from build123d import *

# Parameters (mm, degrees)
BOSS_EXTRUDE1_DEPTH     = 5
CUT_EXTRUDE1_DEPTH      = 5
CUT_EXTRUDE1_DEPTH_BACK = 10
SKETCH2_R               = 1.4
FILLET1_R               = 10
FILLET2_R               = 0.5
CUT_EXTRUDE3_DEPTH      = 7
SKETCH6_W               = 4.5
SKETCH6_H               = 5
BOSS_EXTRUDE2_DEPTH     = 0.5
SKETCH7_W               = 9
SKETCH7_H               = 1
BOSS_EXTRUDE3_DEPTH     = 5
BOSS_EXTRUDE4_DEPTH     = 5
CUT_EXTRUDE5_START      = 5
SKETCH11_R              = 4.1
CUT_EXTRUDE5_DEPTH      = 5
CUT_EXTRUDE7_DEPTH      = 5
FILLET3_R               = 10


with BuildPart() as part:
    # Sketch1 → Boss-Extrude1 (new body)
    with BuildSketch(Plane(origin=(0, 0, 0), x_dir=(1, 0, 0), z_dir=(0, 1, 0))):
        Polygon((0, 0), (0, 9), (40, 9), (40, 0), (24, 0), (24, 5), (16, 5), (16, 0), align=None)
    extrude(amount=BOSS_EXTRUDE1_DEPTH)

    # Sketch2 → Cut-Extrude1 (cut, two sides: drawn at the far end of the back side and taken through both)
    with BuildSketch(Plane(origin=(0, 5, 0), x_dir=(1, 0, 0), z_dir=(0, 1, 0)).offset(-CUT_EXTRUDE1_DEPTH_BACK)):
        with Locations(Location((8, 6, 0), (0, 0, 270))):
            Circle(SKETCH2_R)
        with Locations(Location((32, 6, 0), (0, 0, 270))):
            Circle(SKETCH2_R)
        Polygon((5, 3.7), (0, 3.7), (0, 1), align=None)
        Polygon((13, 1), (8, 3.7), (3, 1), align=None)
        Polygon((16, 3.7), (11, 3.7), (16, 1), align=None)
        Polygon((24, 3.7), (24, 1), (29, 3.7), align=None)
        Polygon((32, 3.7), (27, 1), (37, 1), align=None)
        Polygon((40, 3.7), (35, 3.7), (40, 1), align=None)
    extrude(amount=CUT_EXTRUDE1_DEPTH + CUT_EXTRUDE1_DEPTH_BACK, mode=Mode.SUBTRACT)

    # Fillet1
    fillet1_edges = [part.edges().sort_by_distance(p)[0] for p in [
        (32, 2.5, -3.7),
        (8, 2.5, -3.7),
    ]]
    fillet(fillet1_edges, radius=FILLET1_R)

    # Fillet2
    fillet2_edges = [part.edges().sort_by_distance(p)[0] for p in [
        (0, 2.5, 0),
        (0, 2.5, -9),
        (40, 2.5, -9),
        (40, 2.5, 0),
        (24, 2.5, 0),
        (24, 2.5, -5),
        (16, 2.5, -5),
        (16, 2.5, 0),
        (0, 2.5, -1),
        (0, 2.5, -3.7),
        (16, 2.5, -3.7),
        (16, 2.5, -1),
        (24, 2.5, -3.7),
        (24, 2.5, -1),
        (40, 2.5, -3.7),
        (40, 2.5, -1),
    ]]
    fillet(fillet2_edges, radius=FILLET2_R)

    # Sketch4 → Cut-Extrude3 (cut)
    with BuildSketch(Plane(origin=(0, 5, 0), x_dir=(1, 0, 0), z_dir=(0, 1, 0))):
        Polygon((10.483197095, 1), (8, 2.335141884), (5.076146091, 1.898147599), (11, 3.7), (16.021662669, 1), align=None)
        Polygon((29.516802905, 1), (32, 2.335141884), (34.923853909, 1.898147599), (29, 3.7), (23.978337331, 1), align=None)
    extrude(amount=-CUT_EXTRUDE3_DEPTH, mode=Mode.SUBTRACT)

    # Sketch6 → Boss-Extrude2 (add)
    with BuildSketch(Plane.XY.offset(-3.7)):
        with Locations((13.25, 2.5)):
            Rectangle(SKETCH6_W, SKETCH6_H)
        with Locations((26.75, 2.5)):
            Rectangle(SKETCH6_W, SKETCH6_H)
    boss_extrude2 = extrude(amount=BOSS_EXTRUDE2_DEPTH)

    # Mirror1: Boss-Extrude2 across plane
    add(boss_extrude2.mirror(Plane.XY.offset(-2.35)))

    # Sketch7 → Boss-Extrude3 (add)
    with BuildSketch(Plane(origin=(0, 5, 0), x_dir=(1, 0, 0), z_dir=(0, 1, 0))):
        with Locations((20, 0.5)):
            Rectangle(SKETCH7_W, SKETCH7_H)
    extrude(amount=-BOSS_EXTRUDE3_DEPTH)

    # Sketch9 → Boss-Extrude4 (add)
    with BuildSketch(Plane(origin=(0, 5, 0), x_dir=(1, 0, 0), z_dir=(0, 1, 0))):
        with BuildLine():
            ThreePointArc((16.02382093, 1), (20, 4.1), (23.97617907, 1))
            Line((23.97617907, 1), (24.5, 1))
            Line((24.5, 1), (24.5, 1.5))
            ThreePointArc((24.5, 1.5), (20, 4.74341649), (15.5, 1.5))
            Line((15.5, 1.5), (15.5, 1))
            Line((15.5, 1), (16.02382093, 1))
        make_face()
    extrude(amount=-BOSS_EXTRUDE4_DEPTH)

    # Sketch11 → Cut-Extrude5 (cut)
    with BuildSketch(Plane(origin=(0, 0, 0), x_dir=(1, 0, 0), z_dir=(0, 1, 0)).offset(CUT_EXTRUDE5_START)):
        with Locations((20, 0)):
            Circle(SKETCH11_R)
    extrude(amount=-CUT_EXTRUDE5_DEPTH, mode=Mode.SUBTRACT)

    # Sketch10 → Cut-Extrude7 (cut)
    with BuildSketch(Plane(origin=(0, 5, 0), x_dir=(1, 0, 0), z_dir=(0, 1, 0))):
        with BuildLine():
            ThreePointArc((15.5, 3.7), (20, 6.85), (24.5, 3.7))
            ThreePointArc((24.5, 3.7), (24.146446609, 3.846446609), (24, 4.2))
            Line((24, 4.2), (24, 4.5))
            ThreePointArc((24, 4.5), (23.853553391, 4.853553391), (23.5, 5))
            Line((23.5, 5), (16.5, 5))
            ThreePointArc((16.5, 5), (16.146446609, 4.853553391), (16, 4.5))
            Line((16, 4.5), (16, 4.2))
            ThreePointArc((16, 4.2), (15.853553391, 3.846446609), (15.5, 3.7))
        make_face()
        with BuildLine():
            Line((24.963087063, 3.7), (24.5, 3.7))
            Line((24.5, 3.7), (24.5, 3.2))
            Line((24.5, 3.2), (25.072694865, 3.2))
            ThreePointArc((25.072694865, 3.2), (25.02411482, 3.451364366), (24.963087063, 3.7))
        make_face()
        with BuildLine():
            Line((15.5, 3.2), (15.5, 3.7))
            Line((15.5, 3.7), (15.036912937, 3.7))
            ThreePointArc((15.036912937, 3.7), (14.97588518, 3.451364366), (14.927305135, 3.2))
            Line((14.927305135, 3.2), (15.5, 3.2))
        make_face()
        with BuildLine():
            Line((15.5, 3.7), (16.031107798, 3.7))
            Line((16.031107798, 3.7), (16.5, 5))
            ThreePointArc((16.5, 5), (16.146446609, 4.853553391), (16, 4.5))
            Line((16, 4.5), (16, 4.2))
            ThreePointArc((16, 4.2), (15.853553391, 3.846446609), (15.5, 3.7))
        make_face()
        with BuildLine():
            Line((24.195310158, 3.7), (24.5, 3.7))
            ThreePointArc((24.5, 3.7), (24.146446609, 3.846446609), (24, 4.2))
            Line((24, 4.2), (24, 4.5))
            ThreePointArc((24, 4.5), (23.853553391, 4.853553391), (23.5, 5))
            Line((23.5, 5), (23.319457032, 5))
            Line((23.319457032, 5), (24.195310158, 3.7))
        make_face()
    extrude(amount=-CUT_EXTRUDE7_DEPTH, mode=Mode.SUBTRACT)

    # Fillet3
    # the kernel refuses this fillet: 10 mm, written as the material it takes off along each edge
    with BuildSketch(Plane(origin=(15.5, 8.6255598, -3.7), x_dir=(-1, 0, 0), z_dir=(0, -1, 0))) as fillet3_piece_1:
        with BuildLine():
            CenterArc((7.243737761, 7.350018783), FILLET3_R, 217.432435618, 9.874939203)
            Line((-0.696968767, 1.271764112), (-0.855782897, 1.150199019))
            ThreePointArc((-0.855782897, 1.150199019), (-0.475456762, 0.566296996), (-0.187919463, -0.068456376))
            Line((-0.187919463, -0.068456376), (0, -0.2))
            ThreePointArc((0, -0.2), (0.231543531, -0.2), (0.327474049, -0.147000376))
            Line((0.327474049, -0.147000376), (0.463087063, 0))
        make_face()
    extrude(amount=12.251119601, mode=Mode.SUBTRACT)
    with BuildSketch(Plane(origin=(24.5, 8.6255598, -3.7), x_dir=(-0.4805938979656583, 0, -0.8769432736717777), z_dir=(0, -1, 0))) as fillet3_piece_2:
        with BuildLine():
            CenterArc((2.964253367, 9.884721283), FILLET3_R, 251.41682279, 9.874939203)
            Line((-0.222556817, 0.406101085), (-0.28629302, 0.216528681))
            ThreePointArc((-0.28629302, 0.216528681), (-0.286667063, 0.106931763), (-0.175388655, -0.09611878))
            Line((-0.175388655, -0.09611878), (0.030280589, -0.197694426))
            ThreePointArc((0.030280589, -0.197694426), (0.72511196, -0.144789729), (1.419943331, -0.197694426))
            Line((1.419943331, -0.197694426), (1.45022392, 0))
        make_face()
    extrude(amount=12.251119601, mode=Mode.SUBTRACT)


solid = part.part
Geometry: final body of the model. Coordinates: model frame, mm. A direction names the side the tool comes from. Give positions to 0.01 mm unless a question says otherwise; leave off trailing zeros. Write each loop counter-clockwise with the first axis right and the second up, starting at its lowest first coordinate (ties: lowest second). Pieces come first, ordered by that corner, then holes. Notation, with made-up numbers: (-36.75, 83) -> (-1.75, 83) arc R20 ccw to (-1.75, 102) -> close; hole circle Ø10 at (63, 27.25). An arc over 180 degrees is marked (long way). Answer as a JSON object with one key per item and string values.
1. Mould query, pull axis X, two halves, no side actions, for faces 4 (the flat face through (19.72, 0, -4.56)), 5 (the flat face through (13, 3, -1.5)), 6 (the flat face through (40, 2, -6)). Classes: pulls with the +X half, pulls with the -X half, needs draft (parallel to the pull), parting line crosses it, or undercut.
Ans:
{"face 4": "needs draft", "face 5": "undercut", "face 6": "pulls with the +X half"}
2. Cut plane A-A on z = -2.75. Output: boundary loops of the cut face in (x, y).
Ans:
{"outline": "(3.24, 0) -> (7.88, 0) -> (7.88, 5) -> (3.24, 5) -> close; (16.14, 0) -> (16.96, 0) -> (16.96, 5) -> (16.14, 5) -> close; (23.04, 0) -> (23.86, 0) -> (23.86, 5) -> (23.04, 5) -> close; (32.12, 0) -> (36.76, 0) -> (36.76, 5) -> (32.12, 5) -> close"}
3. Cut plane D-D on y = 3.9. Count the separate pieces of the cut face and the enclosed holes in it, and give its area (3 significant figures).
Ans:
{"separate pieces": "1", "enclosed holes": "3", "area": "249 mm^2"}
4. Ray query, probe 1 along Z at (x, y) = (32, 2.9); probe 2 along Z at (x, y) = (27.5, 0.8); probe 3 along X at (y, z) = (3, -7). Return the intervals inside material, ascending. Write a range as from..to.
Ans:
{"probe 1": "z = -9..-7.4, -4.6..-2.79, -1..0", "probe 2": "z = -9..-3.2, -1.5..0", "probe 3": "x = 0..7.02, 8.98..31.02, 32.98..40"}
5. Cut plane C-C on x = 18.5. Output: boundary loops of the cut face in (y, z).
Ans:
{"outline": "(0, -9) -> (5, -9) -> (5, -6.61) -> (0, -6.61) -> close; (0, -4.5) -> (5, -4.5) -> (5, -3.82) -> (0, -3.82) -> close"}
6. Access query for faces 1 (the flat face through (37.336, 2.465, -2.439)), 2 (the flat face through (31.99, 2.54, -2.79)), 3 (the flat face through (8, 3, 0)). Directions: +Z, -Z, +X, -X, +Y, -Y. A direction counts if a zero-diameter tool reaches every point of the face in a straight line with its end or side. Return the directions, or none.
Ans:
{"face 1": "+X, +Y, -Y", "face 2": "+Y, -Y", "face 3": "+Z, +X, -X, +Y, -Y"}
7. Cut plane B-B on x = 8. Output: boundary loops of the cut face in (y, z), and give its area (3 significant figures).
Ans:
{"outline": "(0, -9) -> (5, -9) -> (5, -7.4) -> (0, -7.4) -> close; (0, -4.6) -> (5, -4.6) -> (5, -2.79) -> (0, -2.79) -> close; (0, -1) -> (5, -1) -> (5, 0) -> (0, 0) -> close", "area": "22.1 mm^2"}
